Verification items for the finished model (mm, model axes). Face numbers are marked on the shaded views. A direction names the side the tool comes from. Coordinates: 2 decimals unless noted, no trailing zeros. Order: outer loops, then holes, each group sorted by start corner. A loop starts at its lowest first (then second) coordinate and runs counter-clockwise, first axis right, second up. Notation, with made-up numbers: (78, 12) - (89, 12) arc R25 ccw to (89, 46) - close; hole circle Ø10 at (33, -11). An arc over 180 degrees is marked (long way). One line per question, with ' | ' between items. Start each with the question number.
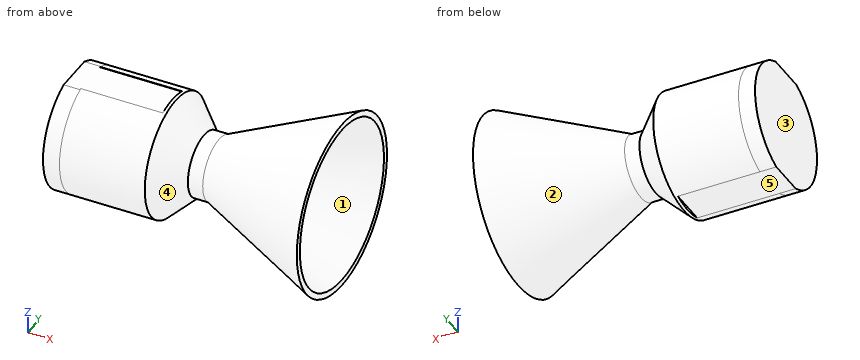
from build123d import *

# Parameters (mm, degrees)
SCALE1_SCALE        = 3
SKETCH5_W           = 6.092075514
SKETCH5_H           = 37.994626104
SKETCH5_W_2         = 6.963088047
CUT_EXTRUDE1_DEPTH  = 213.004502745
SCALE2_SCALE        = 0.6
BOSS_EXTRUDE1_DEPTH = 10


with BuildPart() as part:
    # Sketch1 → Revolve1 (revolve)
    with BuildSketch(Plane.XY, mode=Mode.PRIVATE) as revolve1_sk:
        Polygon((84.678634707, 29.475453574), (84.678634707, 27.468448008), (43.302663782, 8.644223267), (37.73625143, 8.644223267), (28.722559742, 17.657914956), (0, 17.657914956), (0, 20.25452291), (28.722559742, 20.25452291), (38.298141584, 10.678941067), (43.302663782, 10.678941067), align=None)
    revolve(revolve1_sk.sketch.rotate(Axis((0, 0, 0), (1, 0, 0)), 90), axis=Axis((0, 0, 0), (1, 0, 0)))


with BuildPart() as part_1:
    # Scale1: scaled about (41.420833763, 0, 0)
    add(part.part.scale(SCALE1_SCALE).moved(Location((-82.841667526, 0, 0))))

    # Sketch5 → Cut-Extrude1 (cut, through all)
    with BuildSketch(Plane(origin=(0, 0, 0), x_dir=(0, 0, -1), z_dir=(1, 0, 0))):
        with Locations((60.76356873, 0)):
            Rectangle(SKETCH5_W, SKETCH5_H)
        with Locations((-60.763568731, 0)):
            Rectangle(SKETCH5_W_2, SKETCH5_H)
    extrude(amount=-CUT_EXTRUDE1_DEPTH, mode=Mode.SUBTRACT)


with BuildPart() as part_2:
    # Scale2: scaled about (43.48021303, 0, -0.13779422)
    add(part_1.part.scale(SCALE2_SCALE).moved(Location((17.392085212, 0, -0.055117688))))

    # Sketch6 → Boss-Extrude1 (add)
    with BuildSketch(Plane.ZY.offset(32.312915304)):
        with BuildLine():
            Line((-34.685636272, 11.398387831), (-34.685636272, -11.398387831))
            ThreePointArc((-34.685636272, -11.398387831), (-0.459415669, -36.455899464), (34.314097136, -12.163598765))
            Line((34.314097136, -12.163598765), (34.314097136, -11.398387831))
            Line((34.314097136, -11.398387831), (34.314097136, 11.398387831))
            Line((34.314097136, 11.398387831), (34.314097136, 12.163598765))
            ThreePointArc((34.314097136, 12.163598765), (-0.459415669, 36.455899464), (-34.685636272, 11.398387831))
        make_face()
    extrude(amount=BOSS_EXTRUDE1_DEPTH)


solid = part_2.part
Item 1: Section check D-D (x = 23). Record the cut outline in (y, z), then the cut area to 3 significant figures.
Item 2: Mould release check, pull along Z, two halves, no side actions. Record for the marked faces 1, 2 and 3: +Z half, -Z half, draft (parallel to the pull), parting line (faces both ways), or undercut.
Item 3: Set-up check for the marked faces 4 and 5: record each of +Z, -Z, +X, -X, +Y, -Y from which the full face is reachable in a straight line by a thin tool's end or side.
Item 4: Gauge pin test, flat ends, axial feed: pin 1 (7 mm diameter, centred on x = -19.5, y = -4.5, fed in from -Z); pin 2 (7.5 mm diameter, centred on x = -25, y = -1, fed in from +Z); pin 3 (18.5 mm diameter, centred on y = 0, z = -0.06, fed in from +X). Record the tip position at first contact, or that the pin passes through.
Item 5: Section check B-B (y = 0). Record the cut outline in (x, z), then the cut area to 3 significant figures.
Item 6: Thickness scan on probe 1 along X at (y, z) = (-12, 29); probe 2 along X at (y, z) = (24.5, -7); probe 3 along X at (y, z) = (-3, 15). Record the ranges inside material, lowest first. Write a range as from..to.
Item 7: Section check C-C (y = -24.5). Give the number of separate pieces and of enclosed holes in the cut face, then the cut area to 3 significant figures.
Item 8: Section check A-A (x = -7). Record the cut outline in (y, z).
Completed:
1) outline: circle Ø65.69 at (0, -0.06); hole circle Ø56.34 at (0, -0.06) | area: 896 mm^2
2) face 1: undercut | face 2: parting line | face 3: draft
3) face 4: none | face 5: -Z, -X, +Y, -Y
4) pin 1: stops at z = -34.69 | pin 2: stops at z = 34.31 | pin 3: stops at x = -32.31
5) outline: (-42.31, -34.69) - (17.39, -34.69) - (17.39, -36.51) - (19.39, -36.51) - (36.62, -19.28) - (45.63, -19.28) - (120.11, -53.11) - (120.11, -49.5) - (45.63, -15.61) - (35.61, -15.61) - (19.39, -31.84) - (-32.31, -31.84) - (-32.31, 31.73) - (19.39, 31.73) - (35.61, 15.5) - (45.63, 15.5) - (120.11, 49.39) - (120.11, 53) - (45.63, 19.17) - (36.62, 19.17) - (19.39, 36.4) - (17.39, 36.4) - (17.39, 34.31) - (-42.31, 34.31) - close | area: 1,750 mm^2
6) probe 1: x = -42.31..-32.31, 19.74..24.41, 72.52..80.53 | probe 2: x = -42.31..-32.31, 25.71..30.38, 59.37..67.4 | probe 3: x = -42.31..-32.31
7) separate pieces: 2 | enclosed holes: 1 | area: 2,180 mm^2
8) outline: (-11.4, -34.69) - (11.4, -34.69) arc R36.46 ccw to (11.4, 34.58) - (11.4, 34.31) - (-11.4, 34.31) - (-11.4, 34.58) arc R36.46 ccw to start; hole circle Ø63.57 at (0, -0.06)
